Geometry: final body of the model. Coordinates: model frame, mm. Face numbers are marked on the shaded views. A direction names the side the tool comes from. Give positions to 0.01 mm unless a question says otherwise; leave off trailing zeros. Loops run counter-clockwise (first coordinate to the right, second up) from the corner with the lowest first, then second, coordinate; pieces in that order, holes last. Notation, with made-up numbers: (73.5, -30.75) -> (87.5, -30.75) arc R24 cw to (87.5, -17.75) -> close; hole circle Ø3 at (-6.75, -17). An arc over 180 degrees is marked (long way). Answer in a Markdown table with one row per item. Add a question column.
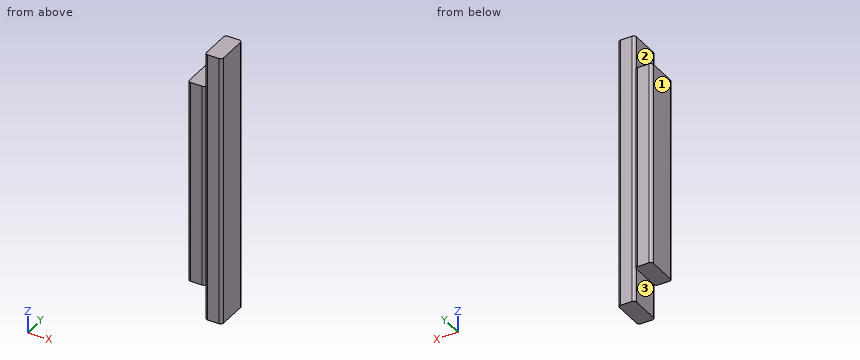
from build123d import *

# Parameters (mm, degrees)
F1_DEPTH = 304.8
F2_DEPTH = 266.7
F3_DEPTH = 38.1


# Not quite as in the source:
# - a feature names something its author has since deleted; it is built from what else it names


with BuildPart() as f1:
    # F0 (on Top) → F1 (new body)
    with BuildSketch(Plane.XY):
        with BuildLine():
            Line((19.05, 34.9504), (19.05, 3.1496))
            ThreePointArc((19.05, 3.1496), (19.972496482, 0.922496482), (22.1996, 0))
            Line((22.1996, 0), (34.9504, 0))
            ThreePointArc((34.9504, 0), (37.177503518, 0.922496482), (38.1, 3.1496))
            Line((38.1, 3.1496), (38.1, 34.9504))
            ThreePointArc((38.1, 34.9504), (37.177503518, 37.177503518), (34.9504, 38.1))
            Line((34.9504, 38.1), (22.1996, 38.1))
            ThreePointArc((22.1996, 38.1), (19.972496482, 37.177503518), (19.05, 34.9504))
        make_face()
    extrude(amount=F1_DEPTH)

    # F0 (on Top) → F2 (join)
    with BuildSketch(Plane.XY):
        with BuildLine():
            ThreePointArc((0, 3.1496), (0.922496482, 0.922496482), (3.1496, 0))
            Line((3.1496, 0), (15.9004, 0))
            ThreePointArc((15.9004, 0), (18.127503518, 0.922496482), (19.05, 3.1496))
            Line((19.05, 3.1496), (19.05, 34.9504))
            ThreePointArc((19.05, 34.9504), (18.127503518, 37.177503518), (15.9004, 38.1))
            Line((15.9004, 38.1), (3.1496, 38.1))
            ThreePointArc((3.1496, 38.1), (0.922496482, 37.177503518), (0, 34.9504))
            Line((0, 34.9504), (0, 3.1496))
        make_face()
        with BuildLine():
            Line((19.05, 34.9504), (19.05, 3.1496))
            ThreePointArc((19.05, 3.1496), (19.972496482, 0.922496482), (22.1996, 0))
            Line((22.1996, 0), (34.9504, 0))
            ThreePointArc((34.9504, 0), (37.177503518, 0.922496482), (38.1, 3.1496))
            Line((38.1, 3.1496), (38.1, 34.9504))
            ThreePointArc((38.1, 34.9504), (37.177503518, 37.177503518), (34.9504, 38.1))
            Line((34.9504, 38.1), (22.1996, 38.1))
            ThreePointArc((22.1996, 38.1), (19.972496482, 37.177503518), (19.05, 34.9504))
        make_face()
    extrude(amount=F2_DEPTH)

    # F0 (on Top) → F3 (cut)
    with BuildSketch(Plane.XY):
        with BuildLine():
            ThreePointArc((0, 3.1496), (0.922496482, 0.922496482), (3.1496, 0))
            Line((3.1496, 0), (15.9004, 0))
            ThreePointArc((15.9004, 0), (18.127503518, 0.922496482), (19.05, 3.1496))
            Line((19.05, 3.1496), (19.05, 34.9504))
            ThreePointArc((19.05, 34.9504), (18.127503518, 37.177503518), (15.9004, 38.1))
            Line((15.9004, 38.1), (3.1496, 38.1))
            ThreePointArc((3.1496, 38.1), (0.922496482, 37.177503518), (0, 34.9504))
            Line((0, 34.9504), (0, 3.1496))
        make_face()
    extrude(amount=F3_DEPTH, mode=Mode.SUBTRACT)


solid = f1.part
(1) Pin query (flat end, axial travel): pin 1 Ø4 at (x, y) = (15.5, 25) entering from -Z; pin 2 Ø6 at (x, y) = (8, 24) entering from +Z; pin 3 Ø16 at (y, z) = (15.5, 13.5) entering from -X. Return the tip coordinate at first contact, or that it passes through.
(2) Reachability of the marked faces 1, 2 and 3 from +Z, -Z, +X, -X, +Y, -Y: full face, straight path, thin tool, end or side. Return the list, or none.
(3) Material intervals for line 1 along Z through (x, y) = (15, 6.5); line 2 along X through (y, z) = (31.5, 275); line 3 along Y through (x, z) = (16.5, 223), sorted ascending. Write a range as from..to.
(4) Cut plane A-A on z = 284. Return the cut outline in (x, y).
(5) Cut plane B-B on y = 6. Return the cut outline in (x, z), then the cut area to 3 significant figures.
(6) Cut plane C-C on x = 12. Return the cut outline in (y, z), then the cut area to 3 significant figures.
Answer list:
| question | item | result |
|---|---|---|
| 1 | pin 1 | stops at z = 38.1 |
| 1 | pin 2 | stops at z = 266.7 |
| 1 | pin 3 | stops at x = 19.05 |
| 2 | face 1 | +Z, -Z, -X, +Y, -Y |
| 2 | face 2 | +Z, -X, +Y, -Y |
| 2 | face 3 | -Z, -X, +Y, -Y |
| 3 | line 1 | z = 38.1..266.7 |
| 3 | line 2 | x = 19.05..38.1 |
| 3 | line 3 | y = 0.06..38.04 |
| 4 | outline | (19.05, 3.15) arc R3.15 ccw to (22.2, 0) -> (34.95, 0) arc R3.15 ccw to (38.1, 3.15) -> (38.1, 34.95) arc R3.15 ccw to (34.95, 38.1) -> (22.2, 38.1) arc R3.15 ccw to (19.05, 34.95) -> close |
| 5 | outline | (0, 38.1) -> (19.05, 38.1) -> (19.05, 0) -> (38.1, 0) -> (38.1, 304.8) -> (19.05, 304.8) -> (19.05, 266.7) -> (0, 266.7) -> close |
| 5 | area | 10,200 mm² |
| 6 | outline | (0, 38.1) -> (38.1, 38.1) -> (38.1, 266.7) -> (0, 266.7) -> close |
| 6 | area | 8,710 mm² |
